Source: CAD feature listing. Evaluate the final solid. Frame: model axes, mm. A direction names the side the tool comes from. Give positions to 0.01 mm unless a question says otherwise; leave off trailing zeros. Loops run counter-clockwise (first coordinate to the right, second up) from the corner with the lowest first, then second, coordinate; pieces in that order, holes last. Notation, with made-up numbers: (-30, 88.5) - (12, 88.5) arc R26 ccw to (12, 110.5) - close; hole circle Ø9 at (70, -26). An arc over 180 degrees is marked (long way). Put each result on its own line as item: value.
```python
from build123d import *

# Parameters (mm, degrees)
F0_R     = 7.5
F1_DEPTH = 500
F3_DEPTH = 35.001


with BuildPart() as f1:
    # F0 (on Top) → F1 (new body)
    with BuildSketch(Plane.XY):
        with BuildLine():
            Line((-155, 0), (-17.5, 0))
            ThreePointArc((-17.5, 0), (-12.3743686708, -12.3743686708), (0, -17.5))
            Line((0, -17.5), (155, -17.5))
            Line((155, -17.5), (155, 0))
            Line((155, 0), (17.5, 0))
            ThreePointArc((17.5, 0), (12.3743686708, 12.3743686708), (0, 17.5))
            Line((0, 17.5), (-155, 17.5))
            Line((-155, 17.5), (-155, 0))
        make_face()
        Circle(F0_R, mode=Mode.SUBTRACT)
    extrude(amount=F1_DEPTH)

    # F2 (on face) → F3 (cut, through all)
    with BuildSketch(Plane.XZ.offset(17.5)):
        Polygon((-17.5, 450), (-130, 450), (-130, 50), (-17.5, 50), (0, 50), (130, 50), (130, 450), (0, 450), align=None)
    extrude(amount=-F3_DEPTH, mode=Mode.SUBTRACT)


solid = f1.part
```
1) Access query for faces 1 (the flat face through (-130, 9, 253)), 2 (the flat face through (2, -8, 450)), 3 (the flat face through (-133, 0, 246)), 4 (the flat face through (-135, 17.5, 249)), 5 (the flat face through (133, 0, 246)). Directions: +Z, -Z, +X, -X, +Y, -Y. A direction counts if a zero-diameter tool reaches every point of the face in a straight line with its end or side. Return the directions, or none.
Check result:
face 1: +X, +Y, -Y
face 2: +Y, -Y
face 3: +Z, -Z, -X, -Y
face 4: +Z, -Z, +X, -X, +Y
face 5: +Z, -Z, +X, +Y
2) Section query A-A, the plane z = 136.5. Output: boundary loops of the cut face in (x, y).
Check result:
outline: (-155, 0) - (-130, 0) - (-130, 17.5) - (-155, 17.5) - close; (130, -17.5) - (155, -17.5) - (155, 0) - (130, 0) - close
3) Material intervals for line 1 along Z through (x, y) = (-112, 4.5); line 2 along X through (y, z) = (6, 193); line 3 along Y through (x, z) = (47, 470.5), sorted ascending. Write a range as [from, to].
Check result:
line 1: [0, 50], [450, 500]
line 2: [-155, -130]
line 3: [-17.5, 0]
4) Section query B-B, the plane x = -93. Output: boundary loops of the cut face in (y, z), plus the area to 3 significant figures.
Check result:
outline: (0, 0) - (17.5, 0) - (17.5, 50) - (0, 50) - close; (0, 450) - (17.5, 450) - (17.5, 500) - (0, 500) - close
area: 1,750 mm²
5) Mould query, pull axis Z, two halves, no side actions, for faces 6 (the cylindrical face through (-7.493, 0.33, 474.65)), 7 (the flat face through (130, -9, 247)), 8 (the flat face through (-2, 8, 0)). Classes: pulls with the +Z half, pulls with the -Z half, needs draft (parallel to the pull), parting line crosses it, or undercut.
Check result:
face 6: needs draft
face 7: undercut
face 8: pulls with the -Z half
6) Pin query (flat end, axial travel): P1, Ø3, axis at y = 11.5, z = 82, coming from the +X side; P2, Ø12, axis at x = 0, y = 0, coming from the -Z side; P3, Ø19, axis at y = -13, z = 248, coming from the -X side. Return the tip coordinate at first contact, or that it passes through.
Check result:
P1: x = -130
P2: through
P3: x = 130
